Autodesk Inventor part; units mm, degrees
ref_plane "YZ Plane" through (0, 0, 0) normal (1, 0, 0) x (0, 1, 0)
ref_plane "XZ Plane" through (0, 0, 0) normal (0, 1, 0) x (-1, 0, 0)
ref_plane "XY Plane" through (0, 0, 0) normal (0, 0, 1) x (1, 0, 0)
sketch "Sketch1" plane through (0, 0, 0) normal (0, 0, 1) x (1, 0, 0)
  line L0 (0, 0) -> (25.4, 0)
  line L1 (25.4, 0) -> (25.4, 25.4)
  line L2 (25.4, 25.4) -> (0, 25.4)
  line L3 (0, 25.4) -> (0, 0)
  line L4 (1.5875, 1.5875) -> (23.8125, 1.5875)
  line L5 (23.8125, 1.5875) -> (23.8125, 23.8125)
  line L6 (23.8125, 23.8125) -> (1.5875, 23.8125)
  line L7 (1.5875, 23.8125) -> (1.5875, 1.5875)
  dimension "d0" = 25.4
  dimension "d1" = 25.4
  dimension "d2" = 1.5875
extrude "Extrusion1" add sketch "Sketch1" along normal mid plane 685.8
properties part number "SUP_005_Middle ConnectorBar" material "Aluminum 6061"
CAD build for the part. Positions are in the model's coordinates, mm. A direction names the side the tool comes from. Coordinates: 2 decimals unless noted, no trailing zeros. Loops run counter-clockwise (first coordinate to the right, second up) from the corner with the lowest first, then second, coordinate; pieces in that order, holes last. Notation, with made-up numbers: (-14.75, -8.5) -> (28.25, -8.5) arc R13 cw to (28.25, -0.5) -> close; hole circle Ø9 at (-11, 35.25). An arc over 180 degrees is marked (long way). One line per item, written item: value.
1. Flat gauge pin, fed straight in: P1, Ø5, axis at x = 19, y = 21, coming from the +Z side. Where does the tip first touch, or does it go through?
Answers:
P1: passes through
2. Slice it at A-A on y = 10.25. Write the cut outline in (x, z).
Answers:
outline: (0, -342.9) -> (1.59, -342.9) -> (1.59, 342.9) -> (0, 342.9) -> close; (23.81, -342.9) -> (25.4, -342.9) -> (25.4, 342.9) -> (23.81, 342.9) -> close
3. Drill centre line: line 1 (X direction, y = 4.5, z = -271.5). Where is it in solid material? Low to high. Write a range as [from, to].
Answers:
line 1: x = [0, 1.59], [23.81, 25.4]
4. Slice it at C-C on z = 159. Write the cut outline in (x, y).
Answers:
outline: (0, 0) -> (25.4, 0) -> (25.4, 25.4) -> (0, 25.4) -> close; hole (1.59, 1.59) -> (23.81, 1.59) -> (23.81, 23.81) -> (1.59, 23.81) -> close
5. Pull direction X, two halves, no side cores. Call faces 3 (the face through (13, 25.4, -5)), 4 (the face through (13, 23.812, -5)), 5 (the face through (25.4, 13, -5)): pulls with the +X half, pulls with the -X half, needs draft (parallel to the pull), parting line crosses it, or undercut.
Answers:
face 3: needs draft
face 4: undercut
face 5: pulls with the +X half
6. Which spindle directions (+Z, -Z, +X, -X, +Y, -Y) get a long thin tool onto all of the face, cutting with end or side? Do faces 1 (the face through (13, 1.588, -5)), 2 (the face through (1, 13, -342.9)). Say none if no direction does.
Answers:
face 1: +Z, -Z
face 2: -Z, +X, -X, +Y, -Y
